```python
from build123d import *

# Parameters (mm, degrees)
SKETCH1_R           = 12.51
SKETCH1_R_2         = 4.01
BOSS_EXTRUDE1_DEPTH = 2
FILLET1_R           = 4.25
CUT_EXTRUDE1_REACH  = 4
SKETCH2_R           = 2.25


with BuildPart() as part:
    # Sketch1 → Boss-Extrude1 (new body)
    with BuildSketch(Plane.XY):
        with BuildLine():
            ThreePointArc((-26.243645437, 38.5), (-53.422989473, 40.673842303), (-57.51289283, 13.716189899))
            Line((-57.51289283, 13.716189899), (-54.973496399, 10))
            Line((-54.973496399, 10), (-85, 10))
            Line((-85, 10), (-85, -10))
            Line((-85, -10), (-41.306829732, -10))
            Line((-41.306829732, -10), (-10.556829732, -55))
            Line((-10.556829732, -55), (10.805406659, -55))
            Line((10.805406659, -55), (41.391170475, -10))
            Line((41.391170475, -10), (85, -10))
            Line((85, -10), (85, 10))
            Line((85, 10), (54.984843282, 10))
            Line((54.984843282, 10), (57.38463841, 13.530753113))
            ThreePointArc((57.38463841, 13.530753113), (53.511141019, 40.603568515), (26.243645437, 38.5))
            Line((26.243645437, 38.5), (-26.243645437, 38.5))
        make_face()
        with Locations((0, -35)):
            Circle(SKETCH1_R, mode=Mode.SUBTRACT)
        with Locations((-75, 0)):
            Circle(SKETCH1_R_2, mode=Mode.SUBTRACT)
        with Locations((-41, 25)):
            Circle(SKETCH1_R, mode=Mode.SUBTRACT)
        with Locations((75, 0)):
            Circle(SKETCH1_R_2, mode=Mode.SUBTRACT)
        with Locations((41, 25)):
            Circle(SKETCH1_R, mode=Mode.SUBTRACT)
    extrude(amount=BOSS_EXTRUDE1_DEPTH)

    # Fillet1
    fillet1_edges = [part.edges().sort_by_distance(p)[0] for p in [
        (-85, -10, 1),
        (-85, 10, 1),
        (85, -10, 1),
        (85, 10, 1),
        (54.984843282, 10, 1),
        (-54.973496399, 10, 1),
        (41.391170475, -10, 1),
        (-41.306829732, -10, 1),
        (26.243645437, 38.5, 1),
        (-26.243645437, 38.5, 1),
    ]]
    fillet(fillet1_edges, radius=FILLET1_R)

    # Sketch2 → Cut-Extrude1 (cut, up to next)
    with BuildSketch(Plane.XY.offset(2), mode=Mode.PRIVATE) as cut_extrude1_sk1:
        with Locations((-41, 41.5)):
            Circle(SKETCH2_R)
    cut_extrude1_tool1 = extrude(cut_extrude1_sk1.sketch, amount=-CUT_EXTRUDE1_REACH, mode=Mode.PRIVATE) & part.part
    add(cut_extrude1_tool1.solids().sort_by_distance((-41, 41.5, 2))[0], mode=Mode.SUBTRACT)
    # Sketch2 → Cut-Extrude1 (cut, up to next)
    with BuildSketch(Plane.XY.offset(2), mode=Mode.PRIVATE) as cut_extrude1_sk2:
        with Locations((-41, 8.5)):
            Circle(SKETCH2_R)
    cut_extrude1_tool2 = extrude(cut_extrude1_sk2.sketch, amount=-CUT_EXTRUDE1_REACH, mode=Mode.PRIVATE) & part.part
    add(cut_extrude1_tool2.solids().sort_by_distance((-41, 8.5, 2))[0], mode=Mode.SUBTRACT)
    # Sketch2 → Cut-Extrude1 (cut, up to next)
    with BuildSketch(Plane.XY.offset(2), mode=Mode.PRIVATE) as cut_extrude1_sk3:
        with Locations((-16.5, -35)):
            Circle(SKETCH2_R)
    cut_extrude1_tool3 = extrude(cut_extrude1_sk3.sketch, amount=-CUT_EXTRUDE1_REACH, mode=Mode.PRIVATE) & part.part
    add(cut_extrude1_tool3.solids().sort_by_distance((-16.5, -35, 2))[0], mode=Mode.SUBTRACT)
    # Sketch2 → Cut-Extrude1 (cut, up to next)
    with BuildSketch(Plane.XY.offset(2), mode=Mode.PRIVATE) as cut_extrude1_sk4:
        with Locations((16.5, -35)):
            Circle(SKETCH2_R)
    cut_extrude1_tool4 = extrude(cut_extrude1_sk4.sketch, amount=-CUT_EXTRUDE1_REACH, mode=Mode.PRIVATE) & part.part
    add(cut_extrude1_tool4.solids().sort_by_distance((16.5, -35, 2))[0], mode=Mode.SUBTRACT)
    # Sketch2 → Cut-Extrude1 (cut, up to next)
    with BuildSketch(Plane.XY.offset(2), mode=Mode.PRIVATE) as cut_extrude1_sk5:
        with Locations((41, 8.5)):
            Circle(SKETCH2_R)
    cut_extrude1_tool5 = extrude(cut_extrude1_sk5.sketch, amount=-CUT_EXTRUDE1_REACH, mode=Mode.PRIVATE) & part.part
    add(cut_extrude1_tool5.solids().sort_by_distance((41, 8.5, 2))[0], mode=Mode.SUBTRACT)
    # Sketch2 → Cut-Extrude1 (cut, up to next)
    with BuildSketch(Plane.XY.offset(2), mode=Mode.PRIVATE) as cut_extrude1_sk6:
        with Locations((41, 41.5)):
            Circle(SKETCH2_R)
    cut_extrude1_tool6 = extrude(cut_extrude1_sk6.sketch, amount=-CUT_EXTRUDE1_REACH, mode=Mode.PRIVATE) & part.part
    add(cut_extrude1_tool6.solids().sort_by_distance((41, 41.5, 2))[0], mode=Mode.SUBTRACT)


solid = part.part
```
Model file for the job. Use its own axes, mm. Round coordinates to 2 decimals unless told otherwise and drop trailing zeros. Order: outer loops, then holes, each group sorted by start corner. A loop starts at its lowest first (then second) coordinate and runs counter-clockwise, first axis right, second up. Notation, with made-up numbers: (-19.75, 25) -> (3.25, 25) arc R9 cw to (3.25, 37) -> close; hole circle Ø9 at (37, 82). An arc over 180 degrees is marked (long way). Use one line per item in the form item = value.
Item 1: Flat gauge pins, fed straight in: pin 1 Ø3 at (x, y) = (55, -10) entering from -Z; pin 2 Ø0.6 at (x, z) = (-69, 1.5) entering from -Y; pin 3 Ø0.6 at (x, z) = (-10.5, 1) entering from +Y; pin 4 Ø1 at (x, z) = (-69.5, 1.5) entering from +Y. Where does each tip first touch, or does it go through?
Returned:
pin_1 = 0
pin_2 = -10
pin_3 = 38.5
pin_4 = 10
Item 2: Cut at B-B, the plane y = 0. Write the cut outline in (x, z).
Returned:
outline = (-85, 0) -> (-79.01, 0) -> (-79.01, 2) -> (-85, 2) -> close; (-70.99, 0) -> (70.99, 0) -> (70.99, 2) -> (-70.99, 2) -> close; (79.01, 0) -> (85, 0) -> (85, 2) -> (79.01, 2) -> close
Item 3: Drill centre lines: line 1 (Y direction, x = 41, z = 1.65); line 2 (Y direction, x = 0, z = 0.45); line 3 (X direction, y = 6.5, z = 1.75). Where is each one in solid material? Low to high.
Returned:
line_1 = -10.92 to 6.25, 10.75 to 12.49, 37.51 to 39.25, 43.75 to 45
line_2 = -55 to -47.51, -22.49 to 38.5
line_3 = -84.93 to -42.03, -39.97 to 39.97, 42.03 to 84.93
Item 4: Cut at D-D, the plane y = 25. Write the cut outline in (x, z).
Returned:
outline = (-61, 0) -> (-53.51, 0) -> (-53.51, 2) -> (-61, 2) -> close; (-28.49, 0) -> (28.49, 0) -> (28.49, 2) -> (-28.49, 2) -> close; (53.51, 0) -> (61, 0) -> (61, 2) -> (53.51, 2) -> close
Item 5: Cut at C-C, the plane x = -75. Write the cut outline in (y, z), and give its area (3 significant figures).
Returned:
outline = (-10, 0) -> (-4.01, 0) -> (-4.01, 2) -> (-10, 2) -> close; (4.01, 0) -> (10, 0) -> (10, 2) -> (4.01, 2) -> close
area = 24.0 mm^2
Item 6: Cut at A-A, the plane x = 0. Write the cut outline in (y, z), and give its area (3 significant figures).
Returned:
outline = (-55, 0) -> (-47.51, 0) -> (-47.51, 2) -> (-55, 2) -> close; (-22.49, 0) -> (38.5, 0) -> (38.5, 2) -> (-22.49, 2) -> close
area = 137 mm^2
Item 7: Pull direction Y, two halves, no side cores. Call faces 1 (the face through (25.26, -33.73, 0.99)), 2 (the face through (38.752, 8.599, 1.014)), 3 (the face through (-1, 7, 0)): released by +Y, released by -Y, zero draft, split by the parting line, or undercut.
Returned:
face_1 = released by -Y
face_2 = undercut
face_3 = zero draft
